Verification items for the finished model (mm, model axes). A direction names the side the tool comes from. Give positions to 0.01 mm unless a question says otherwise; leave off trailing zeros. Write each loop counter-clockwise with the first axis right and the second up, starting at its lowest first coordinate (ties: lowest second). Pieces come first, ordered by that corner, then holes. Notation, with made-up numbers: M 77,62 L 86,62 A30 cw 86,99 Z; hole C 56,20 d5. An arc over 180 degrees is marked long. Write item = value, one per line.
from build123d import *

# Parameters (mm, degrees)
F0_W            = 6.096
F0_H            = 1.778
F1_DEPTH        = 7.62
F2_R            = 1.5
F3_DEPTH        = 1.905
F3_COPIES_COUNT = 3
F4_R            = 5.08
F5_R            = 0.508


# Not quite as in the source:
# - a pattern or mirror of a feature is missing from the dataset's text; its kind, count and spacing are read off the source's solid


with BuildPart() as f1:
    # F0 (on Top) → F1 (new body)
    with BuildSketch(Plane.XY):
        Polygon((10.9985226281, 0), (5.499261314, 9.525), (-5.499261314, 9.525), (-10.9985226281, 0), (-5.499261314, -9.525), (5.499261314, -9.525), align=None)
        with BuildLine():
            ThreePointArc((3.048, 0.889), (3.1430896424, 0.4490128061), (3.175, 0))
            ThreePointArc((3.175, 0), (3.1430896424, -0.4490128061), (3.048, -0.889))
            ThreePointArc((3.048, -0.889), (0, -3.175), (-3.048, -0.889))
            ThreePointArc((-3.048, -0.889), (-3.175, 0), (-3.048, 0.889))
            ThreePointArc((-3.048, 0.889), (0, 3.175), (3.048, 0.889))
        make_face(mode=Mode.SUBTRACT)
        Rectangle(F0_W, F0_H)
        with BuildLine():
            Line((-3.048, -0.889), (-3.048, 0.889))
            ThreePointArc((-3.048, 0.889), (-3.175, 0), (-3.048, -0.889))
        make_face()
        with BuildLine():
            ThreePointArc((3.048, -0.889), (3.1430896424, -0.4490128061), (3.175, 0))
            ThreePointArc((3.175, 0), (3.1430896424, 0.4490128061), (3.048, 0.889))
            Line((3.048, 0.889), (3.048, -0.889))
        make_face()
    extrude(amount=F1_DEPTH)

    # F2 (on Right) → F3 (join, symmetric)
    with BuildSketch(Plane.YZ):
        with BuildLine():
            Line((-9.525, 7.62), (-3.985, 7.62))
            Line((-3.985, 7.62), (-3.985, 11.43))
            ThreePointArc((-3.985, 11.43), (-6.755, 14.2), (-9.525, 11.43))
            Line((-9.525, 11.43), (-9.525, 7.62))
        make_face()
        with Locations((-6.755, 11.43)):
            Circle(F2_R, mode=Mode.SUBTRACT)
    f3 = extrude(amount=F3_DEPTH, both=True)

    # F3_copies: F3 ×3 about axis
    f3_copies_axis = Axis((0, 0, 0), (0, 0, 1))
    for i in range(1, F3_COPIES_COUNT):
        add(f3.rotate(f3_copies_axis, i * 360 / F3_COPIES_COUNT))

    # F4
    f4_edges = [f1.edges().sort_by_distance(p)[0] for p in [
        (-5.499261, -9.525, 3.81),
        (-10.998523, 0, 3.81),
        (-5.499261, 9.525, 3.81),
        (5.499261, 9.525, 3.81),
        (10.998523, 0, 3.81),
        (5.499261, -9.525, 3.81),
    ]]
    fillet(f4_edges, radius=F4_R)

    # F5
    f5_edges = [f1.edges().sort_by_distance(p)[0] for p in [
        (0, -0.889, 7.62),
        (0, 0.889, 7.62),
        (0, -0.889, 0),
        (0, 0.889, 0),
        (0, 3.175, 0),
        (-8.248892, 4.7625, 0),
        (8.248892, 4.7625, 0),
        (10.212644, 0, 0),
        (5.106322, 8.844409, 0),
        (8.248892, -4.7625, 0),
        (0, 9.525, 0),
        (5.106322, -8.844409, 0),
        (-5.106322, 8.844409, 0),
        (0, -9.525, 0),
        (-5.106322, -8.844409, 0),
        (-10.212644, 0, 0),
        (-8.248892, -4.7625, 0),
        (0, -3.175, 0),
    ]]
    fillet(f5_edges, radius=F5_R)


solid = f1.part
1) Depth check by flat-ended pin: P1, Ø1, axis at y = 1.5, z = 8, coming from the -X side; P2, Ø4, axis at x = -7, z = 3.5, coming from the +Y side; P3, Ø2, axis at y = -3.5, z = 4.5, coming from the +X side. Enter the tip coordinate at first touch or a pass-through.
From the geometry:
P1 = -10.07
P2 = 8.9
P3 = 9.55
2) Tool access check on faces 1 (the flat face through (1.905, -7, 9)), 2 (the cylindrical face through (5.8, 3.4, 14.2)), 3 (the flat face through (4.931, 5.047, 9.494)), 4 (the flat face through (0, 0.889, 4)), 5 (the flat face through (6.84, 1.75, 9.49)). Record the directions out of +Z, -Z, +X, -X, +Y, -Y that give a thin tool (end or side, any length) a straight path to the whole face; none if there is none.
From the geometry:
face_1 = +Z, +X, +Y, -Y
face_2 = +Z
face_3 = +Z, +Y
face_4 = +Z, -Z
face_5 = +Z, +X, -Y
3) Cross-section at B-B on x = -0.75. Count the separate pieces of the cut face and the enclosed holes in it, plus the area to 3 significant figures.
From the geometry:
separate_pieces = 3
enclosed_holes = 1
area = 137 mm^2
4) Cross-section at A-A on z = 4.75. Record the boundary of the cut face in (x, y) (3 decimals).
From the geometry:
outline = M -9.532,-2.54 L -6.966,-6.985 A5.08 ccw -2.566,-9.525 L 2.566,-9.525 A5.08 ccw 6.966,-6.985 L 9.532,-2.54 A5.08 ccw 9.532,2.54 L 6.966,6.985 A5.08 ccw 2.566,9.525 L -2.566,9.525 A5.08 ccw -6.966,6.985 L -9.532,2.54 A5.08 ccw Z; hole M -3.048,-0.889 A3.175 ccw 3.048,-0.889 Z; hole M -3.048,0.889 L 3.048,0.889 A3.175 ccw Z
5) Material ranges on probe 1 along Y at (x, z) = (1.75, 4.25) (3 decimals); probe 2 along X at (y, z) = (-0.25, 6.25); probe 3 along Z at (x, y) = (-3.5, 7.25), recorded low to high. Write a range as from..to.
From the geometry:
probe_1 = -9.525..-2.649, -0.889..0.889, 2.649..9.525
probe_2 = -10.21..10.21
probe_3 = 0..7.62
6) Draft check along Z on faces 6 (the flat face through (-6.84, 1.75, 9.49)), 7 (the cylindrical face through (-5.8, 3.3, 14.2)), 8 (the cylindrical face through (-0.027, -7.945, 10.517)), 9 (the flat face through (0, 0, 0)). Enter one of: +Z half, -Z half, draft (parallel to the pull), parting line (faces both ways), or undercut.
From the geometry:
face_6 = draft
face_7 = +Z half
face_8 = undercut
face_9 = -Z half
